```python
from build123d import *

# Parameters (mm, degrees)
F0_W     = 26.555576
F0_H     = 26.555576
F0_R     = 9.525
F1_DEPTH = 8.6995
F2_R     = 3.175
F3_R     = 11.1125
F4_DEPTH = 7.112
F5_R     = 1.35255
F6_DEPTH = 4.7625


with BuildPart() as f1:
    # F0 (on Top) → F1 (new body)
    with BuildSketch(Plane.XY):
        Rectangle(F0_W, F0_H)
        Circle(F0_R, mode=Mode.SUBTRACT)
    extrude(amount=F1_DEPTH)

    # F2
    f2_edges = [f1.edges().sort_by_distance(p)[0] for p in [
        (-13.277788, 13.277788, 4.34975),
        (-13.277788, -13.277788, 4.34975),
        (13.277788, -13.277788, 4.34975),
        (13.277788, 13.277788, 4.34975),
    ]]
    fillet(f2_edges, radius=F2_R)

    # F3 (on face) → F4 (cut)
    with BuildSketch(Plane(origin=(0, 0, 0), x_dir=(1, 0, 0), z_dir=(0, 0, -1))):
        Circle(F3_R)
    extrude(amount=-F4_DEPTH, mode=Mode.SUBTRACT)

    # F5 (on face) → F6 (cut)
    with BuildSketch(Plane(origin=(0, 0, 0), x_dir=(1, 0, 0), z_dir=(0, 0, -1))):
        with Locations((10.102788, 10.102788)):
            Circle(F5_R)
        with Locations((-10.102788, 10.102788)):
            Circle(F5_R)
        with Locations((-10.102788, -10.102788)):
            Circle(F5_R)
        with Locations((10.102788, -10.102788)):
            Circle(F5_R)
    extrude(amount=-F6_DEPTH, mode=Mode.SUBTRACT)


solid = f1.part
```
Read the model definition and answer for the solid it produces. Units are mm, in the model's axes. A direction names the side the tool comes from. Give positions to 0.01 mm unless a question says otherwise; leave off trailing zeros. Order: outer loops, then holes, each group sorted by start corner. A loop starts at its lowest first (then second) coordinate and runs counter-clockwise, first axis right, second up.
(1) For faces 1 (the flat face through (12, 0, 0)), 2 (the cylindrical face through (9.11, -11.02, 2.35)), determine the directions among +Z, -Z, +X, -X, +Y, -Y from which every point of the face is accessible in a straight line to the end or side of a thin tool.
(2) Find section C-C (z = 1.5). Give the number of separate pieces and of enclosed holes in the cut face, plus the area to 3 significant figures.
(3) Find section A-A (x = 0). Give the vertices of the cut face in (y, z) (1 decimal), plus the area to 3 significant figures.
(4) Straight lines are drawn through the part: L1, parallel to X at y = 0, z = 7.85 (3 decimals); L2, parallel to X at y = 0, z = 5.75; L3, parallel to X at y = -11.25, z = 2.75. For each, find the intervals that lie inside material, in ascending order.
(5) Find section D-D (y = 10.5). Give the vertices of the cut face in (x, z), plus the area to 3 significant figures.
(6) Given pin 1 (0.8 mm diameter, centred on x = 10.5, y = -10, fed in from -Z); pin 2 (5 mm diameter, centred on x = 7, y = -2, fed in from -Z), each flat-ended and moving along its own axis, determine where each tip first touches the part or whether it passes through.
(7) For a pull along Y with two mould halves and no side action, classify faces 3 (the flat face through (-5, -8.3, 7.112)), 4 (the cylindrical face through (12.323, -12.372, 4.411)), 5 (the cylindrical face through (-12.372, 12.323, 4.411)), 6 (the flat face through (-10, 10, 4.762)) as released by +Y, released by -Y, zero draft, split by the parting line, or undercut.
Result sheet:
1. face 1: -Z, +X, -X, +Y, -Y
1. face 2: -Z
2. separate pieces: 1
2. enclosed holes: 5
2. area: 286 mm2
3. outline: (-13.3, 0) - (-11.1, 0) - (-11.1, 7.1) - (-9.5, 7.1) - (-9.5, 8.7) - (-13.3, 8.7) - close; (9.5, 7.1) - (11.1, 7.1) - (11.1, 0) - (13.3, 0) - (13.3, 8.7) - (9.5, 8.7) - close
3. area: 42.7 mm2
4. L1: x = -13.278 to -9.525, 9.525 to 13.278
4. L2: x = -13.28 to -11.11, 11.11 to 13.28
4. L3: x = -13.06 to -10.82, -9.39 to 9.39, 10.82 to 13.06
5. outline: (-13.25, 0) - (-11.4, 0) - (-11.4, 4.76) - (-8.81, 4.76) - (-8.81, 0) - (-3.64, 0) - (-3.64, 7.11) - (3.64, 7.11) - (3.64, 0) - (8.81, 0) - (8.81, 4.76) - (11.4, 4.76) - (11.4, 0) - (13.25, 0) - (13.25, 8.7) - (-13.25, 8.7) - close
5. area: 154 mm2
6. pin 1: stops at z = 4.76
6. pin 2: stops at z = 7.11
7. face 3: undercut
7. face 4: released by -Y
7. face 5: released by +Y
7. face 6: undercut
